Check sheet for the modelled part. Datum: model origin and axes. Units: mm. A direction names the side the tool comes from. Round coordinates to 2 decimals unless told otherwise and drop trailing zeros. Write each loop counter-clockwise with the first axis right and the second up, starting at its lowest first coordinate (ties: lowest second). Pieces come first, ordered by that corner, then holes. Notation, with made-up numbers: (-23.5, 86.25) -> (9.5, 86.25) arc R18 cw to (9.5, 118.25) -> close; hole circle Ø10 at (-18.5, 64). An arc over 180 degrees is marked (long way). One line per item, written item: value.
from build123d import *

# Parameters (mm, degrees)
SKETCH1_W           = 16
SKETCH1_H           = 9
BOSS_EXTRUDE1_DEPTH = 3


with BuildPart() as part:
    # Sketch1 → Boss-Extrude1 (new body)
    with BuildSketch(Plane(origin=(0, 0, 0), x_dir=(0, 0, -1), z_dir=(1, 0, 0))):
        Polygon((10, 153.005875518), (20, 153.005875518), (20, 150.005875518), (30, 150.005875518), (30, 153.005875518), (40, 153.005875518), (40, 150.005875518), (50, 150.005875518), (50, 153.005875518), (60, 153.005875518), (60, 150.005875518), (70, 150.005875518), (70, 146.5), (70, 143.5), (70, 140), (73, 140), (73, 130), (70, 130), (70, 120), (73, 120), (73, 110), (70, 110), (70, 100), (73, 100), (73, 90), (70, 90), (70, 83.5), (70, 80), (73, 80), (73, 70), (70, 70), (70, 66.5), (70, 63.5), (70, 60), (73, 60), (73, 50), (70, 50), (70, 40), (73, 40), (73, 30), (70, 30), (70, 20), (73, 20), (73, 10), (70, 10), (70, 6.5), (70, 3.5), (70, 0), (60, 0), (60, -3), (50, -3), (50, 0), (40, 0), (40, -3), (30, -3), (30, 0), (20, 0), (20, -3), (10, -3), (10, 0), (0, 0), (0, 3.5), (5, 3.5), (5, 2.5), (7.5, 2.5), (7.5, 3.5), (16, 3.5), (16, 6.5), (7.5, 6.5), (7.5, 7.5), (5, 7.5), (5, 6.5), (0, 6.5), (0, 10), (-3, 10), (-3, 20), (0, 20), (0, 30), (-3, 30), (-3, 40), (0, 40), (0, 50), (-3, 50), (-3, 60), (0, 60), (0, 63.5), (5, 63.5), (5, 62.5), (7.5, 62.5), (7.5, 63.5), (16, 63.5), (16, 66.5), (7.5, 66.5), (7.5, 67.5), (5, 67.5), (5, 66.5), (0, 66.5), (0, 70), (-3, 70), (-3, 80), (0, 80), (0, 83.5), (5, 83.5), (5, 82.5), (7.5, 82.5), (7.5, 83.5), (16, 83.5), (16, 86.5), (7.5, 86.5), (7.5, 87.5), (5, 87.5), (5, 86.5), (0, 86.5), (0, 90), (-3, 90), (-3, 100), (0, 100), (0, 110), (-3, 110), (-3, 120), (0, 120), (0, 130), (-3, 130), (-3, 140), (0, 140), (0, 143.5), (5, 143.5), (5, 142.5), (7.5, 142.5), (7.5, 143.5), (16, 143.5), (16, 146.5), (7.5, 146.5), (7.5, 147.5), (5, 147.5), (5, 146.5), (0, 146.5), (0, 150.005875518), (10, 150.005875518), align=None)
        with Locations((33.90899457, 144.39356925)):
            Rectangle(SKETCH1_W, SKETCH1_H, mode=Mode.SUBTRACT)
    extrude(amount=BOSS_EXTRUDE1_DEPTH)


solid = part.part
Item 1: Tool access check on faces 4 (the flat face through (1, 105, 0)), 5 (the flat face through (1, 135, -73)), 6 (the flat face through (1, 120, -71)), 7 (the flat face through (1, 152, -60)). Record the directions out of +Z, -Z, +X, -X, +Y, -Y that give a thin tool (end or side, any length) a straight path to the whole face; none if there is none.
Result set:
face 4: +Z, +X, -X
face 5: -Z, +X, -X, +Y, -Y
face 6: -Z, +X, -X
face 7: -Z, +X, -X, +Y
Item 2: Material ranges on line 1 along Y through (x, z) = (0.3, -11); line 2 along Y through (x, z) = (0.85, -29); line 3 along Y through (x, z) = (1.05, -37), recorded low to high.
Result set:
line 1: -3 to 3.5, 6.5 to 63.5, 66.5 to 83.5, 86.5 to 143.5, 146.5 to 153.01
line 2: 0 to 139.89, 148.89 to 150.01
line 3: -3 to 139.89, 148.89 to 153.01
Item 3: Release check for a two-part mould opening along Z. For faces 1 (the flat face through (1, 0, -45)), 2 (the flat face through (1, 75, 3)), 3 (the flat face through (1, 66.5, -3)) record: pulls with the +Z half, pulls with the -Z half, needs draft (parallel to the pull), parting line crosses it, or undercut.
Result set:
face 1: undercut
face 2: pulls with the +Z half
face 3: needs draft
Item 4: Depth check by flat-ended pin: pin 1 (0.9 mm diameter, centred on x = 1.5, y = 47, fed in from -Z); pin 2 (0.8 mm diameter, centred on x = 1, z = -6, fed in from -Y); pin 3 (1.5 mm diameter, centred on x = 1.5, y = 8, fed in from +Z). Enter the tip coordinate at first touch or a pass-through.
Result set:
pin 1: z = -70
pin 2: y = 0
pin 3: z = 0
Item 5: Sectioned sample at B-B (z = -48). Enter the section's corners in (x, y).
Result set:
outline: (0, 0) -> (3, 0) -> (3, 150.01) -> (0, 150.01) -> close
Item 6: Sectioned sample at A-A (y = 43). Enter the section's corners in (x, z), then the cut area to 3 significant figures.
Result set:
outline: (0, -70) -> (3, -70) -> (3, 0) -> (0, 0) -> close
area: 210 mm^2
